from build123d import *

# Parameters (mm, degrees)
F0_R        = 7.5
F1_DEPTH    = 5
F2_R        = 2.8
F3_DEPTH    = 1.5
F4_R        = 3.5
F5_DEPTH    = 3
F6_S5_R     = 2.8
F6_T6_DEPTH = 6
F7_R        = 1.25
F8_DEPTH    = 3.5
F9_R        = 0.6


# Not quite as in the source:
# - a fillet or chamfer that OpenCascade refuses, or shapes differently, is made with other operations: its cross-section is extruded or revolved along the edge and cut away or added
# - two fillets or chamfers of one size are made in one step


with BuildPart() as f1:
    # F0 (on Top) → F1 (new body)
    with BuildSketch(Plane.XY):
        Circle(F0_R)
    extrude(amount=F1_DEPTH)

    # F2 (on face) → F3 (join)
    with BuildSketch(Plane.XY.offset(5)):
        Circle(F2_R)
    extrude(amount=F3_DEPTH)

    # F4 (on face) → F5 (join)
    with BuildSketch(Plane.XY.offset(6.5)):
        Circle(F4_R)
    extrude(amount=F5_DEPTH)

    # F6: chamfer of 1.2 on 2 edges, made by hand


with BuildPart() as f6_tool2:
    # F6_s3 → F6_t4 (revolve)
    with BuildSketch(Plane.XZ):
        Polygon((3.5, 7.7), (2.3, 6.5), (3.5, 6.5), align=None)
    revolve(axis=Axis((0, 0, 6.5), (0, 0, 1)))

    # F6_s5 → F6_t6 (cut, symmetric)
    with BuildSketch(Plane.XY.offset(7.1)):
        Circle(F6_S5_R)
    extrude(amount=F6_T6_DEPTH, both=True, mode=Mode.SUBTRACT)


with BuildPart() as f1_1:
    add(f1.part)

    # F6_t1: cut F6_tool2
    add(f6_tool2.part, mode=Mode.SUBTRACT)

    # F6_s7 → F6_t8 (revolve, cut)
    with BuildSketch(Plane.XZ):
        Polygon((3.5, 8.3), (2.3, 9.5), (3.5, 9.5), align=None)
    revolve(axis=Axis((0, 0, 9.5), (0, 0, 1)), mode=Mode.SUBTRACT)

    # F7 (on face) → F8 (cut)
    with BuildSketch(Plane.XY.offset(9.5)):
        Circle(F7_R)
    extrude(amount=-F8_DEPTH, mode=Mode.SUBTRACT)

    # F9
    f9_edges = [f1_1.edges().sort_by_distance(p)[0] for p in [
        (-1.25, 0, 9.5),
        (-3.5, 0, 8.3),
        (-3.5, 0, 7.7),
        (-7.5, 0, 0),
    ]]
    fillet(f9_edges, radius=F9_R)


solid = f1_1.part
Design review of the part built by this model. Coordinates are the model's own, in mm. A direction names the side the tool comes from. Give positions to 0.01 mm unless a question says otherwise; leave off trailing zeros. Order: outer loops, then holes, each group sorted by start corner. A loop starts at its lowest first (then second) coordinate and runs counter-clockwise, first axis right, second up. Notation, with made-up numbers: (-32, -5) - (-14, -5) arc R14 ccw to (-14, 10) - close; hole circle Ø1 at (44.25, 10). An arc over 180 degrees is marked (long way). Use CSV: the item, a comma, the result in double quotes. Start each with the question number.
Q1. For P1, Ø2, axis at x = -0.5, y = -0.5, coming from the +Z side; P2, Ø5, axis at y = -5, z = 8.5, coming from the +X side; P3, Ø4, axis at x = -3.5, y = 5, coming from the +Z side, all flat-tipped, find the tip position at first contact; note any pin that passes through.
Q2. Machinability: for faces 1 (the face through (0, 0, 6)), 2 (the face through (0, 0, 0)), which of the approach directions +Z, -Z, +X, -X, +Y, -Y give a long, thin tool a straight path to every point of the face, cutting with its end or side? Answer none if there is none.
Q3. Take a section at C-C (z = 9.25). State the section outline as (x, y) points, and give its area (3 significant figures).
Q4. Take a section at A-A (z = 7.25). State the section outline as (x, y) points, and give its area (3 significant figures).
Q5. Draft analysis for pull direction Y (two halves, no side actions). For faces 3 (the face through (-7.493, 0.33, 2.769)), 4 (the face through (3, 0, 5)), 5 (the face through (-0.27, -1.22, 7.47)), state which applies: pulls with the +Y half, pulls with the -Y half, needs draft (parallel to the pull), parting line crosses it, or undercut.
Q6. Take a section at B-B (z = 4.25). State the section outline as (x, y) points, and give its area (3 significant figures).
Q7. For line 1 (Y direction, x = 0, z = 6.7); line 2 (Y direction, x = 0, z = 8.1); line 3 (Z direction, x = -6.5, y = 0.5), list the stretches that pass through material, from the lowest coordinate up.
Calculated:
1,P1,"stops at z = 9.48"
1,P2,"stops at x = 2.41"
1,P3,"stops at z = 5"
2,face 1,"+Z"
2,face 2,"-Z, +X, -X, +Y, -Y"
3,outline,"circle Ø5.1 at (0, 0); hole circle Ø2.73 at (0, 0)"
3,area,"14.6 mm²"
4,outline,"circle Ø6.1 at (0, 0); hole circle Ø2.5 at (0, 0)"
4,area,"24.3 mm²"
5,face 3,"parting line crosses it"
5,face 4,"needs draft"
5,face 5,"undercut"
6,outline,"circle Ø15 at (0, 0)"
6,area,"177 mm²"
7,line 1,"y = -2.8 to -1.25, 1.25 to 2.8"
7,line 2,"y = -3.5 to -1.25, 1.25 to 3.5"
7,line 3,"z = 0 to 5"
